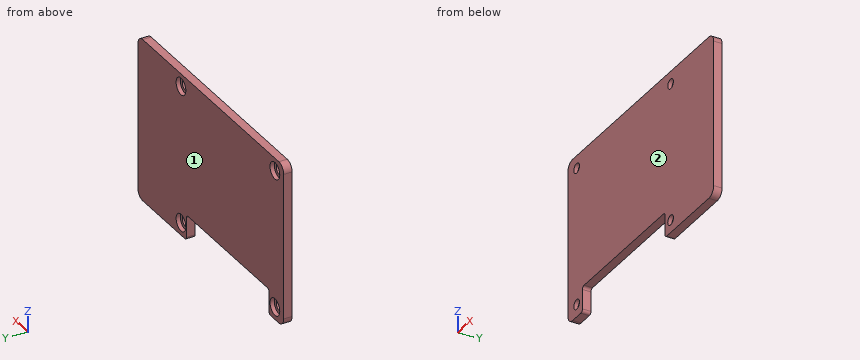
```python
from build123d import *

# Parameters (mm, degrees)
SKETCH1_W           = 90
SKETCH1_H           = 58
BOSS_EXTRUDE1_DEPTH = 3
FILLET1_R           = 3
CUT_EXTRUDE1_REACH  = 55.619
SKETCH2_W           = 51
SKETCH2_H           = 9
FILLET3_R           = 1
CUT_EXTRUDE2_REACH  = 55.619
SKETCH3_R           = 1.75
SKETCH4_R           = 3
CUT_EXTRUDE4_DEPTH  = 1.5


with BuildPart() as part:
    # Sketch1 → Boss-Extrude1 (new body)
    with BuildSketch(Plane(origin=(0, 0, 0), x_dir=(1, 0, 0), z_dir=(0, 1, 0))):
        Rectangle(SKETCH1_W, SKETCH1_H)
    extrude(amount=BOSS_EXTRUDE1_DEPTH)

    # Fillet1
    fillet1_edges = [part.edges().sort_by_distance(p)[0] for p in [
        (-45, 1.5, -29),
        (45, 1.5, -29),
        (45, 1.5, 29),
        (-45, 1.5, 29),
    ]]
    fillet(fillet1_edges, radius=FILLET1_R)

    # Sketch2 → Cut-Extrude1 (cut, up to next)
    with BuildSketch(Plane(origin=(0, 3, 0), x_dir=(1, 0, 0), z_dir=(0, 1, 0)), mode=Mode.PRIVATE) as cut_extrude1_sk1:
        with Locations((-10.5, 24.5)):
            Rectangle(SKETCH2_W, SKETCH2_H)
    cut_extrude1_tool1 = extrude(cut_extrude1_sk1.sketch, amount=-CUT_EXTRUDE1_REACH, mode=Mode.PRIVATE) & part.part
    add(cut_extrude1_tool1.solids().sort_by_distance((-10.5, 3, -24.5))[0], mode=Mode.SUBTRACT)

    # Fillet3
    fillet3_edges = [part.edges().sort_by_distance(p)[0] for p in [
        (-36, 1.5, -20),
        (-36, 1.5, -29),
        (15, 1.5, -29),
        (15, 1.5, -20),
    ]]
    fillet(fillet3_edges, radius=FILLET3_R)

    # Sketch3 → Cut-Extrude2 (cut, up to next)
    with BuildSketch(Plane(origin=(0, 3, 0), x_dir=(1, 0, 0), z_dir=(0, 1, 0)), mode=Mode.PRIVATE) as cut_extrude2_sk1:
        with Locations(Location((-39.6, 24.5, 0), (0, 0, 270))):
            Circle(SKETCH3_R)
    cut_extrude2_tool1 = extrude(cut_extrude2_sk1.sketch, amount=-CUT_EXTRUDE2_REACH, mode=Mode.PRIVATE) & part.part
    # Sketch3 → Cut-Extrude2 (cut, up to next)
    with BuildSketch(Plane(origin=(0, 3, 0), x_dir=(1, 0, 0), z_dir=(0, 1, 0)), mode=Mode.PRIVATE) as cut_extrude2_sk2:
        with Locations(Location((18.4, 24.5, 0), (0, 0, 270))):
            Circle(SKETCH3_R)
    cut_extrude2_tool2 = extrude(cut_extrude2_sk2.sketch, amount=-CUT_EXTRUDE2_REACH, mode=Mode.PRIVATE) & part.part
    cut_extrude2_1 = cut_extrude2_tool1.solids().sort_by_distance((-39.6, 3, -24.5))[0]
    add(cut_extrude2_1, mode=Mode.SUBTRACT)
    cut_extrude2_2 = cut_extrude2_tool2.solids().sort_by_distance((18.4, 3, -24.5))[0]
    add(cut_extrude2_2, mode=Mode.SUBTRACT)
    cut_extrude2 = cut_extrude2_1 + cut_extrude2_2  # Cut-Extrude2 as one shape, for the pattern or mirror that repeats it

    # Mirror1: Cut-Extrude2 across plane
    add(cut_extrude2.mirror(Plane.XY), mode=Mode.SUBTRACT)

    # Sketch4 → Cut-Extrude4 (cut)
    with BuildSketch(Plane(origin=(0, 3, 0), x_dir=(1, 0, 0), z_dir=(0, 1, 0))):
        with Locations(Location((-39.6, 24.5, 0), (0, 0, 270))):
            Circle(SKETCH4_R)
        with Locations(Location((18.4, 24.5, 0), (0, 0, 270))):
            Circle(SKETCH4_R)
    cut_extrude4 = extrude(amount=-CUT_EXTRUDE4_DEPTH, mode=Mode.SUBTRACT)

    # Mirror2: Cut-Extrude4 across plane
    add(cut_extrude4.mirror(Plane.XY), mode=Mode.SUBTRACT)


solid = part.part
```
Could you check a few things on this model? Use its own coordinates, in mm. Face numbers are marked on the shaded views. Round coordinates to 2 decimals unless told otherwise and drop trailing zeros. Loops run counter-clockwise (first coordinate to the right, second up) from the corner with the lowest first, then second, coordinate; pieces in that order, holes last. Notation, with made-up numbers: M -7,29 L 6,29 A33 cw 6,60 Z; hole C -1,-17.5 d7. An arc over 180 degrees is marked long. Put each result on its own line as item: value.
Q1. For pin 1 (3 mm diameter, centred on x = -39.6, z = 24.5, fed in from -Y); pin 2 (1.5 mm diameter, centred on x = -9, y = 1, fed in from -Z); pin 3 (5 mm diameter, centred on x = -39.6, z = 24.5, fed in from +Y), each with a flat end and sliding along its axis, tell me the tip position at first contact or that it passes through.
Check result:
pin 1: through
pin 2: z = -20
pin 3: y = 1.5
Q2. Imagine slicing it at B-B (x = -39.6). Write out the boundary of the cut face in (y, z).
Check result:
outline: M 0,-29 L 3,-29 L 3,-27.5 L 1.5,-27.5 L 1.5,-26.25 L 0,-26.25 Z; M 0,-22.75 L 1.5,-22.75 L 1.5,-21.5 L 3,-21.5 L 3,21.5 L 1.5,21.5 L 1.5,22.75 L 0,22.75 Z; M 0,26.25 L 1.5,26.25 L 1.5,27.5 L 3,27.5 L 3,29 L 0,29 Z
Q3. Imagine slicing it at A-A (z = 24.5). Write out the boundary of the cut face in (x, y).
Check result:
outline: M -45,0 L -41.35,0 L -41.35,1.5 L -42.6,1.5 L -42.6,3 L -45,3 Z; M -37.85,0 L 16.65,0 L 16.65,1.5 L 15.4,1.5 L 15.4,3 L -36.6,3 L -36.6,1.5 L -37.85,1.5 Z; M 20.15,0 L 45,0 L 45,3 L 21.4,3 L 21.4,1.5 L 20.15,1.5 Z
Q4. Thinking about a two-plate mould opening in Y: for the marked faces 1 and 2, which applies, released by +Y, released by -Y, zero draft, split by the parting line, or undercut?
Check result:
face 1: released by +Y
face 2: released by -Y
Q5. Imagine slicing it at D-D (z = -24.5). Write out the boundary of the cut face in (x, y).
Check result:
outline: M -45,0 L -41.35,0 L -41.35,1.5 L -42.6,1.5 L -42.6,3 L -45,3 Z; M -37.85,0 L -36,0 L -36,3 L -36.6,3 L -36.6,1.5 L -37.85,1.5 Z; M 15,0 L 16.65,0 L 16.65,1.5 L 15.4,1.5 L 15.4,3 L 15,3 Z; M 20.15,0 L 45,0 L 45,3 L 21.4,3 L 21.4,1.5 L 20.15,1.5 Z
Q6. Imagine slicing it at C-C (y = 2.1). Write out the boundary of the cut face in (x, z).
Check result:
outline: M -45,-26 A3 ccw -42,-29 L -37,-29 A1 ccw -36,-28 L -36,-21 A1 cw -35,-20 L 14,-20 A1 cw 15,-21 L 15,-28 A1 ccw 16,-29 L 42,-29 A3 ccw 45,-26 L 45,26 A3 ccw 42,29 L -42,29 A3 ccw -45,26 Z; hole C -39.6,-24.5 d6; hole C -39.6,24.5 d6; hole C 18.4,-24.5 d6; hole C 18.4,24.5 d6
Q7. I need wall thicknesses on probe 1 along X at (y, z) = (2.6, -24.5); probe 2 along Z at (x, y) = (-40.5, 0.85); probe 3 along X at (y, z) = (0.7, -24.5). Which ranges of each line are inside material? Lowest first, please.
Check result:
probe 1: -45 to -42.6, -36.6 to -36, 15 to 15.4, 21.4 to 45
probe 2: -29 to -26, -23 to 23, 26 to 29
probe 3: -45 to -41.35, -37.85 to -36, 15 to 16.65, 20.15 to 45
